The listing builds one solid part. Answer for the finished solid, in the listing's coordinates (mm). Face numbers are marked on the shaded views. A direction names the side the tool comes from. Round coordinates to 2 decimals unless told otherwise and drop trailing zeros. Loops run counter-clockwise (first coordinate to the right, second up) from the corner with the lowest first, then second, coordinate; pieces in that order, holes last. Notation, with made-up numbers: (-15, 21.25) - (31, 21.25) arc R13 cw to (31, 38.25) - close; hole circle Ø6 at (56.5, -17). An arc over 180 degrees is marked (long way). Write item = value, one per line. Start each with the question number.
1) Section A-A, the plane x = 0 is taken. Determine the outline of the cut face in (y, z).
2) Straight lines are drawn through the part: line 1 along X through (y, z) = (23.75, -6); line 2 along X through (y, z) = (23.2, -6); line 3 along Z through (x, y) = (0, 26.4). For each, find the intervals that lie inside material, in ascending order.
3) Section D-D, the plane x = 3 is taken. Determine the outline of the cut face in (y, z).
4) A tool of negligible diameter and unlimited length cuts with its end or side. For the marked faces 4, 5, 6 and 7, from which of +Z, -Z, +X, -X, +Y, -Y can it reach the whole face along a straight path? Write none if from no direction.
5) For a pull along X with two mould halves and no side action, classify the marked faces 1, 2 and 3 as released by +X, released by -X, zero draft, split by the parting line, or undercut.
6) Section B-B, the plane z = 0 is taken. Determine the outline of the cut face in (x, y).
7) Section C-C, the plane y = 22.4 is taken. Determine the outline of the cut face in (x, z).
8) Given pin 1 Ø1.5 at (y, z) = (24, 7.5) entering from -X; pin 2 Ø5 at (x, z) = (-1.5, 10) entering from -Y; pin 3 Ø0.8 at (x, z) = (2.5, -12.5) entering from -Y, each flat-ended and moving along its own axis, determine where each tip first touches the part or whether it passes through.
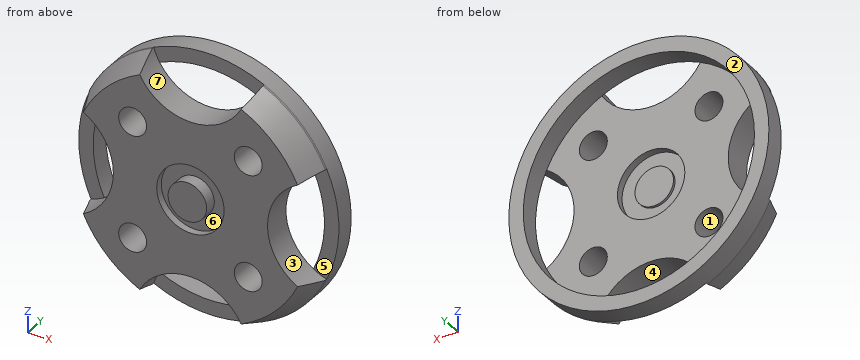
from build123d import *

# Parameters (mm, degrees)
CYLINDER032_R             = 1.45
CYLINDER032_DEPTH         = 10
CYLINDER033_R             = 1.45
CYLINDER033_DEPTH         = 10
CYLINDER034_R             = 1.45
CYLINDER034_DEPTH         = 10
CYLINDER031_R             = 1.45
CYLINDER031_DEPTH         = 10
CYLINDER028_R             = 3.5
CYLINDER028_DEPTH         = 10
CYLINDER026_R             = 6
CYLINDER026_DEPTH         = 10
CYLINDER027_R             = 6
CYLINDER027_DEPTH         = 10
CYLINDER024_R             = 6
CYLINDER024_DEPTH         = 10
CYLINDER025_R             = 6
CYLINDER025_DEPTH         = 10
CYLINDER023_R             = 13.5
CYLINDER023_DEPTH         = 3
CHAMFER003_SIZE2          = 1.2
CHAMFER003_SIZE           = 2.8
CYLINDER010_R             = 12
CYLINDER010_DEPTH         = 2
CYLINDER011_R             = 13.5
CYLINDER011_DEPTH         = 2
CYLINDER030_R             = 2
CYLINDER030_DEPTH         = 3
CYLINDER029_R             = 3.5
CYLINDER029_DEPTH         = 1.5
FUSION008_ROLL_ANGLE      = 90
FUSION008_PLACEMENT_ANGLE = 180


with BuildPart() as cylinder032:
    # Cylinder032 → Cylinder032 (new body)
    with BuildSketch(Plane(origin=(6, -6, 0), x_dir=(1, 0, 0), z_dir=(0, 0, 1))):
        Circle(CYLINDER032_R)
    extrude(amount=CYLINDER032_DEPTH)


with BuildPart() as cylinder033:
    # Cylinder033 → Cylinder033 (new body)
    with BuildSketch(Plane(origin=(-6, -6, 0), x_dir=(1, 0, 0), z_dir=(0, 0, 1))):
        Circle(CYLINDER033_R)
    extrude(amount=CYLINDER033_DEPTH)


with BuildPart() as cylinder034:
    # Cylinder034 → Cylinder034 (new body)
    with BuildSketch(Plane(origin=(-6, 6, 0), x_dir=(1, 0, 0), z_dir=(0, 0, 1))):
        Circle(CYLINDER034_R)
    extrude(amount=CYLINDER034_DEPTH)


with BuildPart() as cylinder031:
    # Cylinder031 → Cylinder031 (new body)
    with BuildSketch(Plane(origin=(6, 6, 0), x_dir=(1, 0, 0), z_dir=(0, 0, 1))):
        Circle(CYLINDER031_R)
    extrude(amount=CYLINDER031_DEPTH)


with BuildPart() as cylinder028:
    # Cylinder028 → Cylinder028 (new body)
    with BuildSketch(Plane.XY):
        Circle(CYLINDER028_R)
    extrude(amount=CYLINDER028_DEPTH)


with BuildPart() as cylinder026:
    # Cylinder026 → Cylinder026 (new body)
    with BuildSketch(Plane(origin=(0, 14, 0), x_dir=(1, 0, 0), z_dir=(0, 0, 1))):
        Circle(CYLINDER026_R)
    extrude(amount=CYLINDER026_DEPTH)


with BuildPart() as cylinder027:
    # Cylinder027 → Cylinder027 (new body)
    with BuildSketch(Plane(origin=(-14, 0, 0), x_dir=(1, 0, 0), z_dir=(0, 0, 1))):
        Circle(CYLINDER027_R)
    extrude(amount=CYLINDER027_DEPTH)


with BuildPart() as cylinder024:
    # Cylinder024 → Cylinder024 (new body)
    with BuildSketch(Plane(origin=(14, 0, 0), x_dir=(1, 0, 0), z_dir=(0, 0, 1))):
        Circle(CYLINDER024_R)
    extrude(amount=CYLINDER024_DEPTH)


with BuildPart() as cylinder025:
    # Cylinder025 → Cylinder025 (new body)
    with BuildSketch(Plane(origin=(0, -14, 0), x_dir=(1, 0, 0), z_dir=(0, 0, 1))):
        Circle(CYLINDER025_R)
    extrude(amount=CYLINDER025_DEPTH)


with BuildPart() as cut022:
    # Cylinder023 → Cylinder023 (new body)
    with BuildSketch(Plane.XY.offset(2)):
        Circle(CYLINDER023_R)
    extrude(amount=CYLINDER023_DEPTH)

    # Chamfer003
    chamfer003_edges = [cut022.edges().sort_by_distance(p)[0] for p in [
        (-13.5, 0, 2),
    ]]
    chamfer003_side = cut022.faces().sort_by_distance((-13.5, 0, 3.5))[0]
    chamfer(chamfer003_edges, length=CHAMFER003_SIZE, length2=CHAMFER003_SIZE2, reference=chamfer003_side)

    # Cut017: cut Cylinder025
    add(cylinder025.part, mode=Mode.SUBTRACT)

    # Cut018: cut Cylinder024
    add(cylinder024.part, mode=Mode.SUBTRACT)

    # Cut019: cut Cylinder027
    add(cylinder027.part, mode=Mode.SUBTRACT)

    # Cut020: cut Cylinder026
    add(cylinder026.part, mode=Mode.SUBTRACT)

    # Cut021: cut Cylinder028
    add(cylinder028.part, mode=Mode.SUBTRACT)


with BuildPart() as cylinder010:
    # Cylinder010 → Cylinder010 (new body)
    with BuildSketch(Plane.XY.offset(5)):
        Circle(CYLINDER010_R)
    extrude(amount=CYLINDER010_DEPTH)


with BuildPart() as stator_full:
    # Cylinder011 → Cylinder011 (new body)
    with BuildSketch(Plane.XY.offset(5)):
        Circle(CYLINDER011_R)
    extrude(amount=CYLINDER011_DEPTH)

    # Cut011: cut Cylinder010
    add(cylinder010.part, mode=Mode.SUBTRACT)

    # Fusion007: union Cut022
    add(cut022.part)

    # Cut022: cut Cylinder031
    add(cylinder031.part, mode=Mode.SUBTRACT)

    # Cut023: cut Cylinder034
    add(cylinder034.part, mode=Mode.SUBTRACT)

    # Cut024: cut Cylinder033
    add(cylinder033.part, mode=Mode.SUBTRACT)

    # Cut025: cut Cylinder032
    add(cylinder032.part, mode=Mode.SUBTRACT)


with BuildPart() as cylinder030:
    # Cylinder030 → Cylinder030 (new body)
    with BuildSketch(Plane.XY.offset(1.5)):
        Circle(CYLINDER030_R)
    extrude(amount=CYLINDER030_DEPTH)


with BuildPart() as stator:
    # Cylinder029 → Cylinder029 (new body)
    with BuildSketch(Plane.XY.offset(2.75)):
        Circle(CYLINDER029_R)
    extrude(amount=CYLINDER029_DEPTH)

    # Fusion006: union Cylinder030
    add(cylinder030.part)

    # Fusion008: union Stator_Full
    add(stator_full.part)


with BuildPart() as stator_1:
    # Fusion008 roll: moved
    add(stator.part.rotate(Axis((0, 0, 0), (1, 0, 0)), FUSION008_ROLL_ANGLE))


with BuildPart() as stator_2:
    # Fusion008 placement: moved
    add(stator_1.part.moved(Location((0, 20, 0))).rotate(Axis((0, 20, 0), (0, 0, 1)), FUSION008_PLACEMENT_ANGLE))


solid = stator_2.part
Geometry check:
q1.outline = (21.5, -2) - (22.75, -2) - (22.75, -3.5) - (22, -3.5) - (22, -8) - (25, -8) - (25, -3.5) - (24.25, -3.5) - (24.25, -2) - (24.5, -2) - (24.5, 2) - (24.25, 2) - (24.25, 3.5) - (25, 3.5) - (25, 8) - (22, 8) - (22, 3.5) - (22.75, 3.5) - (22.75, 2) - (21.5, 2) - close; (25, -13.5) - (27, -13.5) - (27, -12) - (25, -12) - close; (25, 12) - (27, 12) - (27, 13.5) - (25, 13.5) - close
q2.line_1 = -11.59 to -7.45, -4.55 to 4.55, 7.45 to 11.59
q2.line_2 = -11.32 to -7.45, -4.55 to 4.55, 7.45 to 11.32
q2.line_3 = -13.5 to -12, 12 to 13.5
q3.outline = (22, -8.8) - (25, -8.8) - (25, -1.8) - (24.25, -1.8) - (24.25, 1.8) - (25, 1.8) - (25, 8.8) - (22, 8.8) - (22, 1.8) - (22.75, 1.8) - (22.75, -1.8) - (22, -1.8) - close; (25, -13.16) - (27, -13.16) - (27, -11.62) - (25, -11.62) - close; (25, 11.62) - (27, 11.62) - (27, 13.16) - (25, 13.16) - close
q4.face_4 = -Z, -Y
q4.face_5 = +X, -Y
q4.face_6 = -Y
q4.face_7 = +Z, -Y
q5.face_1 = undercut
q5.face_2 = zero draft
q5.face_3 = released by +X
q6.outline = (-13.5, 25) - (-12, 25) - (-12, 27) - (-13.5, 27) - close; (-8, 22) - (-3.5, 22) - (-3.5, 22.75) - (-2, 22.75) - (-2, 21.5) - (2, 21.5) - (2, 22.75) - (3.5, 22.75) - (3.5, 22) - (8, 22) - (8, 25) - (3.5, 25) - (3.5, 24.25) - (2, 24.25) - (2, 24.5) - (-2, 24.5) - (-2, 24.25) - (-3.5, 24.25) - (-3.5, 25) - (-8, 25) - close; (12, 25) - (13.5, 25) - (13.5, 27) - (12, 27) - close
q7.outline = (-11.27, -5.34) arc R12.47 ccw to (-5.34, -11.27) arc R6 cw to (5.34, -11.27) arc R12.47 ccw to (11.27, -5.34) arc R6 cw to (11.27, 5.34) arc R12.47 ccw to (5.34, 11.27) arc R6 cw to (-5.34, 11.27) arc R12.47 ccw to (-11.27, 5.34) arc R6 cw to start; circle Ø4 at (0, 0); hole circle Ø2.9 at (-6, -6); hole circle Ø2.9 at (-6, 6); hole circle Ø7 at (0, 0); hole circle Ø2.9 at (6, -6); hole circle Ø2.9 at (6, 6)
q8.pin_1 = -11.43
q8.pin_2 = 22
q8.pin_3 = 25
